from build123d import *

# Parameters (mm, degrees)
BOSS_EXTRUDE1_DEPTH = 2.5
SKETCH3_R           = 1.27
SKETCH3_W           = 4.75
SKETCH3_H           = 6.5
CUT_EXTRUDE2_DEPTH  = 16.702614432
CUT_EXTRUDE1_START  = -2.5
CUT_EXTRUDE1_DEPTH  = 1.5
SKETCH4_R           = 1.95
CUT_EXTRUDE3_DEPTH  = 1
CUT_EXTRUDE4_START  = -2.5
SKETCH5_W           = 2.71
SKETCH5_H           = 1.15
CUT_EXTRUDE4_DEPTH  = 1


with BuildPart() as part:
    # Sketch1 → Boss-Extrude1 (new body)
    with BuildSketch(Plane(origin=(0, 0, 0), x_dir=(1, 0, 0), z_dir=(0, 1, 0))):
        with BuildLine():
            Line((-10.16, 8.89), (10.16, 8.89))
            ThreePointArc((10.16, 8.89), (11.956051224, 8.146051224), (12.7, 6.35))
            Line((12.7, 6.35), (12.7, -6.35))
            ThreePointArc((12.7, -6.35), (11.956051224, -8.146051224), (10.16, -8.89))
            Line((10.16, -8.89), (-10.16, -8.89))
            ThreePointArc((-10.16, -8.89), (-11.956051224, -8.146051224), (-12.7, -6.35))
            Line((-12.7, -6.35), (-12.7, 6.35))
            ThreePointArc((-12.7, 6.35), (-11.956051224, 8.146051224), (-10.16, 8.89))
        make_face()
    extrude(amount=BOSS_EXTRUDE1_DEPTH)

    # Sketch3 → Cut-Extrude2 (cut, through all)
    with BuildSketch(Plane(origin=(0, 2.5, 0), x_dir=(1, 0, 0), z_dir=(0, 1, 0))):
        with Locations(Location((-10.16, 6.35, 0), (0, 0, 270))):
            Circle(SKETCH3_R)
        with Locations(Location((10.16, 6.35, 0), (0, 0, 270))):
            Circle(SKETCH3_R)
        with Locations(Location((10.16, -6.35, 0), (0, 0, 270))):
            Circle(SKETCH3_R)
        with Locations(Location((-10.16, -6.35, 0), (0, 0, 270))):
            Circle(SKETCH3_R)
        with Locations((10.325, 0)):
            Rectangle(SKETCH3_W, SKETCH3_H)
        with Locations((-10.325, 0)):
            Rectangle(SKETCH3_W, SKETCH3_H)
    extrude(amount=-CUT_EXTRUDE2_DEPTH, mode=Mode.SUBTRACT)

    # Sketch2 → Cut-Extrude1 (cut)
    with BuildSketch(Plane(origin=(0, 2.5, 0), x_dir=(1, 0, 0), z_dir=(0, 1, 0)).offset(CUT_EXTRUDE1_START)):
        with BuildLine():
            Line((-3.81, -5.35), (-3.81, -3.635))
            Line((-3.81, -3.635), (3.31, -3.635))
            Line((3.31, -3.635), (3.31, -5.35))
            Line((3.31, -5.35), (6.486568362, -5.35))
            ThreePointArc((6.486568362, -5.35), (7.036509651, -4.173326382), (7.95, -3.25))
            Line((7.95, -3.25), (12.7, -3.25))
            Line((12.7, -3.25), (12.7, 3.25))
            Line((12.7, 3.25), (7.95, 3.25))
            ThreePointArc((7.95, 3.25), (7.036509651, 4.173326382), (6.486568362, 5.35))
            Line((6.486568362, 5.35), (-7.95, 5.35))
            Line((-7.95, 5.35), (-7.95, 3.25))
            Line((-7.95, 3.25), (-12.7, 3.25))
            Line((-12.7, 3.25), (-12.7, -3.25))
            Line((-12.7, -3.25), (-7.95, -3.25))
            Line((-7.95, -3.25), (-7.95, -5.35))
            Line((-7.95, -5.35), (-3.81, -5.35))
        make_face()
    extrude(amount=CUT_EXTRUDE1_DEPTH, mode=Mode.SUBTRACT)

    # Sketch4 → Cut-Extrude3 (cut)
    with BuildSketch(Plane(origin=(0, 2.5, 0), x_dir=(1, 0, 0), z_dir=(0, 1, 0))):
        with Locations(Location((-10.16, 6.35, 0), (0, 0, 270))):
            Circle(SKETCH4_R)
        with Locations(Location((10.16, 6.35, 0), (0, 0, 270))):
            Circle(SKETCH4_R)
        with Locations(Location((-10.16, -6.35, 0), (0, 0, 270))):
            Circle(SKETCH4_R)
        with Locations(Location((10.16, -6.35, 0), (0, 0, 270))):
            Circle(SKETCH4_R)
    extrude(amount=-CUT_EXTRUDE3_DEPTH, mode=Mode.SUBTRACT)

    # Sketch5 → Cut-Extrude4 (cut)
    with BuildSketch(Plane(origin=(0, 2.5, 0), x_dir=(1, 0, 0), z_dir=(0, 1, 0)).offset(CUT_EXTRUDE4_START)):
        with Locations((-9.305, 3.825)):
            Rectangle(SKETCH5_W, SKETCH5_H)
    extrude(amount=CUT_EXTRUDE4_DEPTH, mode=Mode.SUBTRACT)


solid = part.part
Geometry: final body of the model. Coordinates: model frame, mm. A direction names the side the tool comes from. Round coordinates to 2 decimals unless told otherwise and drop trailing zeros. Order: outer loops, then holes, each group sorted by start corner. A loop starts at its lowest first (then second) coordinate and runs counter-clockwise, first axis right, second up. Notation, with made-up numbers: (7.5, 79) -> (50.5, 79) arc R29 ccw to (50.5, 110) -> close; hole circle Ø5 at (64.5, -38). An arc over 180 degrees is marked (long way). Put each result on its own line as item: value. Start each with the question number.
Q1. Pull-direction query (X, two-part tool) for faces 1 (the flat face through (12.7, 1, 5)), 2 (the flat face through (-7.95, 1, -5)), 3 (the flat face through (0, 2.5, 0)); classes: +X half, -X half, draft (parallel to the pull), parting line (faces both ways), or undercut.
Q2. Reachability of faces 4 (the flat face through (-7.95, 2, 0)), 5 (the cylindrical face through (11.804, 2.007, -5.302)), 6 (the flat face through (-7.95, 1, 4)) from +Z, -Z, +X, -X, +Y, -Y: full face, straight path, thin tool, end or side. Return the list, or none.
Q3. Section D-D on z = -2. Return the cut outline in (x, y), and give its area (3 significant figures).
Q4. First-contact query: pin 1 (1.1 mm diameter, centred on y = 2, z = 0, fed in from +X); pin 2 (3.5 mm diameter, centred on x = 10.16, z = 6.35, fed in from +Y). Flat tips, straight axial feed; report the tip coordinate or a pass-through.
Q5. Section A-A on y = 1.25. Return the cut outline in (x, z) (3 decimals).
Q6. Section B-B on z = 6. Return the cut outline in (x, y), and give its area (3 significant figures).
Q7. Section C-C on x = -3.25. Return the cut outline in (y, z) (3 decimals), and give its area (3 significant figures).
Q8. Line query: probe 1 along X at (y, z) = (2.25, -6.35); probe 2 along X at (y, z) = (0.5, -6.35); probe 3 along Z at (x, y) = (3, 1) (3 decimals). Output: solid intervals per line, ascending.
Ans:
1. face 1: +X half
1. face 2: undercut
1. face 3: draft
2. face 4: -X, +Y, -Y
2. face 5: +Y
2. face 6: -Y
3. outline: (-7.95, 1.5) -> (7.95, 1.5) -> (7.95, 2.5) -> (-7.95, 2.5) -> close
3. area: 15.9 mm2
4. pin 1: stops at x = 7.95
4. pin 2: stops at y = 1.5
5. outline: (-12.7, -6.35) arc R2.54 ccw to (-10.16, -8.89) -> (10.16, -8.89) arc R2.54 ccw to (12.7, -6.35) -> (12.7, -3.25) -> (7.95, -3.25) arc R3.807 ccw to (6.487, -5.35) -> (-7.95, -5.35) -> (-7.95, -3.25) -> (-12.7, -3.25) -> close; (-12.7, 3.25) -> (-7.95, 3.25) -> (-7.95, 5.35) -> (-3.81, 5.35) -> (-3.81, 3.635) -> (3.31, 3.635) -> (3.31, 5.35) -> (6.487, 5.35) arc R3.807 ccw to (7.95, 3.25) -> (12.7, 3.25) -> (12.7, 6.35) arc R2.54 ccw to (10.16, 8.89) -> (-10.16, 8.89) arc R2.54 ccw to (-12.7, 6.35) -> close; hole circle Ø2.54 at (-10.16, -6.35); hole circle Ø2.54 at (-10.16, 6.35); hole circle Ø2.54 at (10.16, -6.35); hole circle Ø2.54 at (10.16, 6.35)
6. outline: (-12.7, 0) -> (-11.38, 0) -> (-11.38, 1.5) -> (-12.08, 1.5) -> (-12.08, 2.5) -> (-12.7, 2.5) -> close; (-8.94, 0) -> (8.94, 0) -> (8.94, 1.5) -> (8.24, 1.5) -> (8.24, 2.5) -> (-8.24, 2.5) -> (-8.24, 1.5) -> (-8.94, 1.5) -> close; (11.38, 0) -> (12.7, 0) -> (12.7, 2.5) -> (12.08, 2.5) -> (12.08, 1.5) -> (11.38, 1.5) -> close
6. area: 48.5 mm2
7. outline: (0, -8.89) -> (2.5, -8.89) -> (2.5, 8.89) -> (0, 8.89) -> (0, 3.635) -> (1.5, 3.635) -> (1.5, -5.35) -> (0, -5.35) -> close
7. area: 31.0 mm2
8. probe 1: x = -12.7 to -12.11, -8.21 to 8.21, 12.11 to 12.7
8. probe 2: x = -12.7 to -11.43, -8.89 to 8.89, 11.43 to 12.7
8. probe 3: z = -8.89 to -5.35, 3.635 to 8.89
